Autodesk Inventor part; units mm, degrees
ref_plane "YZ Plane" through (0, 0, 0) normal (1, 0, 0) x (0, 1, 0)
ref_plane "XZ Plane" through (0, 0, 0) normal (0, 1, 0) x (-1, 0, 0)
ref_plane "XY Plane" through (0, 0, 0) normal (0, 0, 1) x (1, 0, 0)
sketch "スケッチ1" plane through (0, 0, 0) normal (0, 0, 1) x (1, 0, 0)
  line L0 (-100, 100) -> (100, 100)
  line L1 (100, 100) -> (100, -100)
  line L2 (100, -100) -> (-100, -100)
  line L3 (-100, -100) -> (-100, 100)
  line L4 (-100, 100) -> (100, -100) construction
  line L5 (100, 100) -> (-100, -100) construction
  circle A0 centre (0, 0) radius 93.75 construction
  circle A1 centre (-66.2913, 66.2913) radius 4
  circle A2 centre (66.2913, 66.2913) radius 4
  circle A3 centre (66.2913, -66.2913) radius 4
  circle A4 centre (-66.2913, -66.2913) radius 4
  dimension "d0" = 200
  dimension "d1" = 200
  dimension "d2" = 187.5
  dimension "d3" = 8
  dimension "d4" = 8
  dimension "d5" = 8
  dimension "d6" = 8
extrude "押し出し1" add sketch "スケッチ1" along normal blind 3
sketch "スケッチ2" plane through (0, 0, 0) normal (0, 0, -1) x (-1, 0, 0)
  circle A0 centre (0, 0) radius 72.5
  dimension "d9" = 145
extrude "押し出し2" cut sketch "スケッチ2" against normal blind 10
sketch "スケッチ3" plane through (0, 0, 3) normal (0, 0, 1) x (1, 0, 0)
  circle A0 centre (-66.2913, -66.2913) radius 4
  circle A1 centre (66.2913, -66.2913) radius 4
  point P0 (0, 0)
sketch "スケッチ4" plane through (-100, -100, 0) normal (0, -1, 0) x (1, 0, 0)
  line L0 (0, 0) -> (0, 3)
  line L1 (200, 0) -> (200, 3)
  line L2 (0, 3) -> (200, 3)
  line L3 (200, 3) -> (200, 0)
  line L4 (200, 0) -> (0, 0)
  line L5 (0, 0) -> (0, 3)
  point P0 (100, 0)
extrude "押し出し3" add sketch "スケッチ4" along normal blind 50
sketch "スケッチ5" plane through (0, 0, 3) normal (0, 0, 1) x (1, 0, 0)
  circle A0 centre (0, -120) radius 6
  point P0 (0, 0)
  dimension "d14" = 12
extrude "押し出し4" cut sketch "スケッチ5" against normal blind 100
sketch "スケッチ6" plane through (0, 0, 3) normal (0, 0, 1) x (1, 0, 0)
  circle A0 centre (0, -120) radius 6
  line L0 (0, -120) -> (-30, -120)
  line L1 (-30, -120) -> (30, -120)
  line L2 (30, -120) -> (30, -111)
  line L3 (30, -111) -> (30, -129)
  line L4 (30, -129) -> (-30, -111)
  line L5 (-30, -111) -> (-30, -129)
  circle A1 centre (-30, -111) radius 2.5
  circle A2 centre (-30, -129) radius 2.5
  circle A3 centre (30, -111) radius 2.5
  circle A4 centre (30, -129) radius 2.5
  point P0 (0, 0)
  dimension "d17" = 30
  dimension "d18" = 60
  dimension "d19" = 9
  dimension "d20" = 90
  dimension "d21" = 18
  dimension "d22" = 5
  dimension "d23" = 5
  dimension "d24" = 5
  dimension "d25" = 5
extrude "押し出し5" cut sketch "スケッチ6" against normal blind 100 contours A3 | A2 | A1 L5 L4 | L4 L5 A1 | A4 L3 L4 | L4 L3 A4
properties part number "ベアリング板" material "アルミニウム 6061"
CAD build for the part. Positions are in the model's coordinates, mm. Coordinates: 2 decimals unless noted, no trailing zeros. Order: outer loops, then holes, each group sorted by start corner. A loop starts at its lowest first (then second) coordinate and runs counter-clockwise, first axis right, second up.
Item 1: Band-saw the part on D-D on x = -37. List the corners of the cut face in (y, z).
Check sheet entries:
outline: (-150, 0) - (-62.35, 0) - (-62.35, 3) - (-150, 3) - close; (62.35, 0) - (100, 0) - (100, 3) - (62.35, 3) - close
Item 2: Band-saw the part on C-C on z = 0.45. Give the number of separate pieces and of enclosed holes in the cut face, plus the area to 3 significant figures.
Check sheet entries:
separate pieces: 1
enclosed holes: 10
area: 33,100 mm2
Item 3: Band-saw the part on B-B on x = 0. List the corners of the cut face in (y, z).
Check sheet entries:
outline: (-150, 0) - (-126, 0) - (-126, 3) - (-150, 3) - close; (-114, 0) - (-72.5, 0) - (-72.5, 3) - (-114, 3) - close; (72.5, 0) - (100, 0) - (100, 3) - (72.5, 3) - close
Item 4: Two-plate mould, pull along X, no slides. Class faces 1 (the face through (29.67, -108.52, 1.52)), 2 (the face through (-1, -79, 3)), 3 (the face through (63.34, -68.99, 1.48)): +X half, -X half, draft (parallel to the pull), parting line (faces both ways), or undercut.
Check sheet entries:
face 1: undercut
face 2: draft
face 3: undercut
Item 5: Band-saw the part on A-A on y = 0. List the corners of the cut face in (x, z).
Check sheet entries:
outline: (-100, 0) - (-72.5, 0) - (-72.5, 3) - (-100, 3) - close; (72.5, 0) - (100, 0) - (100, 3) - (72.5, 3) - close
Item 6: Drill centre lines: L1, parallel to Y at x = 0, z = 1.95; L2, parallel to X at y = -129, z = 1.45; L3, parallel to Y at x = 30, z = 1.5. Where is each one in solid material? Low to high.
Check sheet entries:
L1: y = -150 to -126, -114 to -72.5, 72.5 to 100
L2: x = -100 to -32.5, -27.5 to 27.5, 32.5 to 100
L3: y = -150 to -131.5, -126.5 to -113.5, -108.5 to -66, 66 to 100
Item 7: Pin check, flat tips, straight feed: pin 1 Ø13 at (x, y) = (66.29, 66.29) entering from +Z; pin 2 Ø9.5 at (x, y) = (0, -120) entering from +Z. Stop position of each tip, or through.
Check sheet entries:
pin 1: stops at z = 3
pin 2: passes through
